from build123d import *

# Parameters (mm, degrees)
SKETCH1_W           = 28
SKETCH1_H           = 20
BOSS_EXTRUDE1_DEPTH = 3
M3_TAPPED_HOLE1_D   = 2.5
SCALE1_SCALE        = 1.5
FILLET1_R           = 2
CHAMFER1_SIZE       = 2


with BuildPart() as part:
    # Sketch1 → Boss-Extrude1 (new body)
    with BuildSketch(Plane(origin=(0, 0, 0), x_dir=(1, 0, 0), z_dir=(0, 1, 0))):
        Rectangle(SKETCH1_W, SKETCH1_H)
    extrude(amount=BOSS_EXTRUDE1_DEPTH)

    # M3 Tapped Hole1 (through all)
    with Locations(Plane(origin=(0, 3, 0), x_dir=(1, 0, 0), z_dir=(0, 1, 0))):
        with Locations((-11, 7), (-11, -7), (10, -7), (10, 7)):
            Hole(M3_TAPPED_HOLE1_D / 2)


with BuildPart() as part_1:
    # Scale1: scaled about (0.018168231, 1.5, 0)
    add(part.part.scale(SCALE1_SCALE).moved(Location((-0.009084115, -0.75, 0))))

    # Fillet1
    fillet1_edges = [part_1.edges().sort_by_distance(p)[0] for p in [
        (20.990915884, 1.5, -15),
        (20.990915884, 1.5, 15),
    ]]
    fillet(fillet1_edges, radius=FILLET1_R)

    # Chamfer1
    chamfer1_edges = [part_1.edges().sort_by_distance(p)[0] for p in [
        (20.990915884, 3.75, 0),
        (-1.009084116, 3.75, -15),
        (20.405129447, 3.75, -14.414213562),
        (20.405129447, 3.75, 14.414213562),
        (-21.009084116, 3.75, 0),
        (-1.009084116, 3.75, 15),
    ]]
    chamfer(chamfer1_edges, length=CHAMFER1_SIZE)


solid = part_1.part
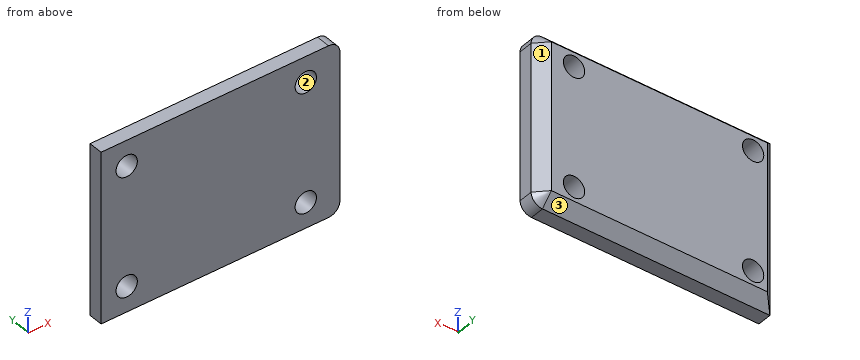
Work out the finished part from the listing and answer in its coordinate system (mm). Face numbers are marked on the shaded views. Give positions to 0.01 mm unless a question says otherwise; leave off trailing zeros. Loops run counter-clockwise (first coordinate to the right, second up) from the corner with the lowest first, then second, coordinate; pieces in that order, holes last. Notation, with made-up numbers: (4, -26) -> (12, -26) arc R8 ccw to (12, -17) -> close; hole circle Ø11 at (85.5, 29.5). An arc over 180 degrees is marked (long way). Use a Markdown table: item, result. Add a question column.
1. Section A-A on z = 10.5 is taken. Determine the outline of the cut face in (x, y), and give its area (3 significant figures).
2. Section B-B on y = 2.2 is taken. Determine the outline of the cut face in (x, z) (3 decimals).
3. Find the intervals of material crossed by probe 1 along X at (y, z) = (1.7, 10.5); probe 2 along Z at (x, y) = (15, 0.2); probe 3 along X at (y, z) = (-0.35, 9.25), in increasing order.
4. Section C-C on x = 14 is taken. Determine the outline of the cut face in (y, z), and give its area (3 significant figures).
5. A flat-ended cylindrical pin translates along its axis: pin 1 Ø3 at (x, z) = (-16.51, 10.5) entering from +Y. Find the tip coordinate at first contact, or state that the pin passes through.
6. Section D-D on x = -5 is taken. Determine the outline of the cut face in (y, z).
7. Determine the mould class of the marked faces 1, 2 and 3 for opening direction Z: released by +Z, released by -Z, zero draft, split by the parting line, or undercut.
Results below:
| question | item | result |
|---|---|---|
| 1 | outline | (-21.01, -0.75) -> (-18.38, -0.75) -> (-18.38, 3.75) -> (-19.01, 3.75) -> (-21.01, 1.75) -> close; (-14.63, -0.75) -> (13.12, -0.75) -> (13.12, 3.75) -> (-14.63, 3.75) -> close; (16.87, -0.75) -> (20.99, -0.75) -> (20.99, 1.75) -> (18.99, 3.75) -> (16.87, 3.75) -> close |
| 1 | area | 151 mm^2 |
| 2 | outline | (-20.559, -14.55) -> (18.991, -14.55) arc R1.55 ccw to (20.541, -13) -> (20.541, 13) arc R1.55 ccw to (18.991, 14.55) -> (-20.559, 14.55) -> close; hole circle Ø3.75 at (-16.509, -10.5); hole circle Ø3.75 at (-16.509, 10.5); hole circle Ø3.75 at (14.991, -10.5); hole circle Ø3.75 at (14.991, 10.5) |
| 3 | probe 1 | x = -21.01 to -18.38, -14.63 to 13.12, 16.87 to 20.99 |
| 3 | probe 2 | z = -15 to -12.37, -8.63 to 8.63, 12.37 to 15 |
| 3 | probe 3 | x = -21.01 to -17.91, -15.11 to 13.59, 16.39 to 20.99 |
| 4 | outline | (-0.75, -15) -> (1.75, -15) -> (3.75, -13) -> (3.75, -12.09) -> (-0.75, -12.09) -> close; (-0.75, -8.91) -> (3.75, -8.91) -> (3.75, 8.91) -> (-0.75, 8.91) -> close; (-0.75, 12.09) -> (3.75, 12.09) -> (3.75, 13) -> (1.75, 15) -> (-0.75, 15) -> close |
| 4 | area | 102 mm^2 |
| 5 | pin 1 | passes through |
| 6 | outline | (-0.75, -15) -> (1.75, -15) -> (3.75, -13) -> (3.75, 13) -> (1.75, 15) -> (-0.75, 15) -> close |
| 7 | face 1 | zero draft |
| 7 | face 2 | undercut |
| 7 | face 3 | released by -Z |
